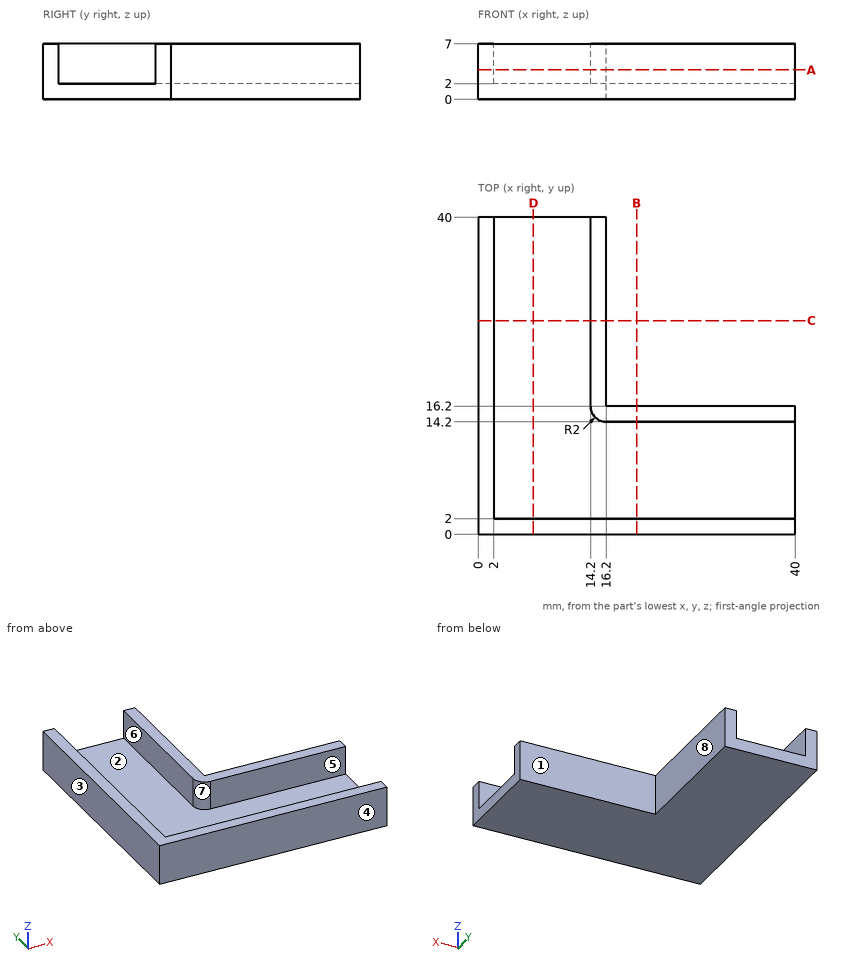
Can you work these out from the drawing? Everything is in mm from the part's minimum corner. A direction names the side the tool comes from. Coordinates: 2 decimals unless noted, no trailing zeros. Loops run counter-clockwise (first coordinate to the right, second up) from the corner with the lowest first, then second, coordinate; pieces in that order, holes last. Notation, with made-up numbers: M -29.75,-33 L -25.75,-33 A11 cw -25.75,-21 Z; hole C -22,-23.75 d6. An arc over 180 degrees is marked long. Put each result on its own line as item: value. Start each with the question number.
(1) Suppose I cut it at B-B on x = 20. Please give me the cut outline in (y, z).
(2) Will this pin go through, and if not, where does the flat tip stop? P1, Ø2.5, axis at y = 18, z = 3.5, coming from the +X side.
(3) Suppose I cut it at D-D on x = 7. Please give me the cut outline in (y, z), then the cut area to 3 significant figures.
(4) For the marked faces 5, 6, 7 and 8, which set-ups out of +Z, -Z, +X, -X, +Y, -Y let a thin tool reach every point of the face, with its end or its side?
(5) Thinking about a two-plate mould opening in Y: for the marked faces 1, 2, 3 and 4, which applies, pulls with the +Y half, pulls with the -Y half, needs draft (parallel to the pull), parting line crosses it, or undercut?
(6) Suppose I cut it at A-A on z = 3.75. Please give me the cut outline in (x, y), then the cut area to 3 significant figures.
(7) I need wall thicknesses on line 1 (X direction, y = 25, z = 5.25); line 2 (Y direction, x = 26.5, z = 1). Which ranges of each line are inside material? Lowest first, please. Write a range as from..to.
Solutions:
1. outline: M 0,0 L 16.2,0 L 16.2,7 L 14.2,7 L 14.2,2 L 2,2 L 2,7 L 0,7 Z
2. P1: stops at x = 16.2
3. outline: M 0,0 L 40,0 L 40,2 L 2,2 L 2,7 L 0,7 Z
3. area: 90.0 mm2
4. face 5: +Z, +X
4. face 6: +Z, +Y
4. face 7: +Z
4. face 8: +Z, -Z, +X, +Y
5. face 1: pulls with the +Y half
5. face 2: undercut
5. face 3: needs draft
5. face 4: pulls with the -Y half
6. outline: M 0,0 L 40,0 L 40,2 L 2,2 L 2,40 L 0,40 Z; M 14.2,16.2 A2 ccw 16.2,14.2 L 40,14.2 L 40,16.2 L 16.2,16.2 L 16.2,40 L 14.2,40 Z
6. area: 254 mm2
7. line 1: x = 0..2, 14.2..16.2
7. line 2: y = 0..16.2
